```python
from build123d import *

# Parameters (mm, degrees)
SKETCH2_R           = 2.996049
BOSS_EXTRUDE1_DEPTH = 7.75
SKETCH3_W           = 9.22
SKETCH3_H           = 15
BOSS_EXTRUDE2_DEPTH = 11.94
BOSS_EXTRUDE3_DEPTH = 5.05
FILLET1_START       = 11.94
FILLET1_DEPTH       = 5.05
SKETCH5_R           = 1.5
CUT_EXTRUDE1_DEPTH  = 7.75
SKETCH6_R           = 2
CUT_EXTRUDE2_DEPTH  = 13.08
CUT_EXTRUDE3_START  = -3
SKETCH7_R           = 3.65
CUT_EXTRUDE3_DEPTH  = 3


with BuildPart() as part:
    # Sketch1 → Revolve1 (revolve)
    with BuildSketch(Plane.XY, mode=Mode.PRIVATE) as revolve1_sk:
        Polygon((0, 3.65), (3, 3.65), (3, 2), (13.08, 2), (13.08, 3.125), (11.941875, 4.08), (5.949776, 4.08), (4.62693, 2.97), (2.16, 5.04), (0, 5.04), align=None)
    revolve(revolve1_sk.sketch.rotate(Axis((-0.163685, 0, 0), (1, 0, 0)), 90), axis=Axis((-0.163685, 0, 0), (1, 0, 0)))

    # Sketch2 → Boss-Extrude1 (add)
    with BuildSketch(Plane.XY):
        with Locations((8.945826, 0)):
            Circle(SKETCH2_R)
    extrude(amount=BOSS_EXTRUDE1_DEPTH)

    # Sketch3 → Boss-Extrude2 (add)
    with BuildSketch(Plane.ZY):
        with Locations((-4.61, 1.5)):
            Rectangle(SKETCH3_W, SKETCH3_H)
    extrude(amount=-BOSS_EXTRUDE2_DEPTH)

    # Sketch4 → Boss-Extrude3 (add)
    with BuildSketch(Plane(origin=(11.94, 0, 0), x_dir=(0, 0, -1), z_dir=(1, 0, 0))):
        Polygon((0, 9), (9.22, 9), (9.22, -6), (7.12, -6), (7.12, 6.9), (0, 6.9), align=None)
    extrude(amount=BOSS_EXTRUDE3_DEPTH)

    # Fillet1: read off the stored shape, not the designer's step
    # Fillet1 outline → Fillet1 (add)
    with BuildSketch(Plane.YZ.offset(FILLET1_START)):
        with BuildLine():
            ThreePointArc((6.9, -2.12), (5.435534, -5.655534), (1.9, -7.12))
            Line((1.9, -7.12), (6.9, -7.12))
            Line((6.9, -7.12), (6.9, -2.12))
        make_face()
    extrude(amount=FILLET1_DEPTH)

    # Chamfer1: read off the stored shape, not the designer's step
    # Chamfer1 outline → Chamfer1 (revolve, cut)
    with BuildSketch(Plane(origin=(8.945826, 0, 0), x_dir=(1, 0, 0), z_dir=(0, -1, 0))):
        Polygon((2.996049, 7.75), (2.496049, 7.75), (2.996049, 7.25), align=None)
    revolve(axis=Axis((8.945826, 0, 0), (0, 0, 1)), mode=Mode.SUBTRACT)

    # Sketch5 → Cut-Extrude1 (cut)
    with BuildSketch(Plane.XY.offset(7.75)):
        with Locations((8.945826, 0)):
            Circle(SKETCH5_R)
    extrude(amount=-CUT_EXTRUDE1_DEPTH, mode=Mode.SUBTRACT)

    # Sketch6 → Cut-Extrude2 (cut)
    with BuildSketch(Plane(origin=(13.08, 0, 0), x_dir=(0, 0, -1), z_dir=(1, 0, 0))):
        with Locations(Location((0, 0, 0), (0, 0, 180))):
            Circle(SKETCH6_R)
    extrude(amount=-CUT_EXTRUDE2_DEPTH, mode=Mode.SUBTRACT)

    # Sketch7 → Cut-Extrude3 (cut)
    with BuildSketch(Plane.ZY.offset(CUT_EXTRUDE3_START)):
        Circle(SKETCH7_R)
    extrude(amount=CUT_EXTRUDE3_DEPTH, mode=Mode.SUBTRACT)


solid = part.part
```
Check sheet for the modelled part. Datum: model origin and axes. Units: mm. A direction names the side the tool comes from. Coordinates: 2 decimals unless noted, no trailing zeros. Loops run counter-clockwise (first coordinate to the right, second up) from the corner with the lowest first, then second, coordinate; pieces in that order, holes last.
1) Gauge pin test, flat ends, axial feed: pin 1 (5 mm diameter, centred on x = 6.5, y = 5, fed in from +Z); pin 2 (3.5 mm diameter, centred on y = 1.5, z = -3, fed in from +X); pin 3 (4.5 mm diameter, centred on y = 0, z = 0, fed in from -X). Record the tip position at first contact, or that the pin passes through.
2) Release check for a two-part mould opening along Y. For faces 1 (the face through (13.08, 2, -1)), 2 (the face through (11.804, 0.9, 5.476)), 3 (the face through (11.94, 0.5, -4.4)) record: released by +Y, released by -Y, zero draft, split by the parting line, or undercut.
3) Sectioned sample at D-D (y = 1.25). Count the separate pieces of the cut face and the enclosed holes in it, and give its area (3 significant figures).
4) Sectioned sample at A-A (x = 12.25). Record the boundary of the cut face in (y, z).
5) Material ranges on probe 1 along Z at (x, y) = (9, -5); probe 2 along X at (y, z) = (3, -4.5); probe 3 along Z at (x, y) = (14.75, -3.5), recorded low to high.
6) Access from +Z, -Z, +X, -X, +Y, -Y to the whole of each face (thin tool, end or side, straight path). Record for faces 4 (the face through (0, 2, -4)), 5 (the face through (3, -2, 2)), 6 (the face through (1.06, 0.11, 5.04)), 7 (the face through (4.84, 0.07, 3.15)).
7) Sectioned sample at B-B (x = 14.5). Record the boundary of the cut face in (y, z).
8) Sectioned sample at C-C (x = 3.75). Record the boundary of the cut face in (y, z).
Check sheet entries:
1. pin 1: stops at z = 3.22
1. pin 2: stops at x = 13.08
1. pin 3: stops at x = 3
2. face 1: zero draft
2. face 2: split by the parting line
2. face 3: undercut
3. separate pieces: 3
3. enclosed holes: 0
3. area: 134 mm2
4. outline: (-6, -9.22) - (9, -9.22) - (9, 0) - (6.9, 0) - (6.9, -2.12) arc R5 cw to (1.9, -7.12) - (-6, -7.12) - close; circle Ø7.64 at (0, 0); hole circle Ø4 at (0, 0)
5. probe 1: z = -9.22 to 0
5. probe 2: x = 0 to 11.94
5. probe 3: z = -9.22 to -7.12
6. face 4: +Z, -Z, -X, +Y, -Y
6. face 5: -X
6. face 6: +Z, -X
6. face 7: +Z
7. outline: (-6, -9.22) - (9, -9.22) - (9, 0) - (6.9, 0) - (6.9, -2.12) arc R5 cw to (1.9, -7.12) - (-6, -7.12) - close
8. outline: (-6, -9.22) - (9, -9.22) - (9, 0) - (3.71, 0) arc R3.71 ccw to (-3.71, 0) - (-6, 0) - close; hole circle Ø4 at (0, 0)
